from build123d import *

# Parameters (mm, degrees)
SKETCH8_W            = 23
SKETCH8_H            = 23
BOSS_EXTRUDE4_DEPTH  = 0.98
SKETCH16_W           = 9.9
SKETCH16_H           = 9.3
BOSS_EXTRUDE11_DEPTH = 0.84
BOSS_EXTRUDE11_TAPER = 20
SKETCH17_R           = 0.522081484
BOSS_EXTRUDE12_DEPTH = 0.1


with BuildPart() as part:
    # Sketch8 → Boss-Extrude4 (new body)
    with BuildSketch(Plane(origin=(0, 0, 0), x_dir=(1, 0, 0), z_dir=(0, 1, 0))):
        Rectangle(SKETCH8_W, SKETCH8_H)
    extrude(amount=BOSS_EXTRUDE4_DEPTH)

    # Sketch16 → Boss-Extrude11 (add)
    with BuildSketch(Plane(origin=(0, 0.98, 0), x_dir=(1, 0, 0), z_dir=(0, 1, 0))):
        Rectangle(SKETCH16_W, SKETCH16_H)
    extrude(amount=BOSS_EXTRUDE11_DEPTH, taper=BOSS_EXTRUDE11_TAPER)

    # Sketch17 → Boss-Extrude12 (add)
    with BuildSketch(Plane(origin=(0, 0.98, 0), x_dir=(1, 0, 0), z_dir=(0, 1, 0))):
        with Locations((-10.659163623, -10.593903438)):
            Circle(SKETCH17_R)
    extrude(amount=BOSS_EXTRUDE12_DEPTH)


solid = part.part
Can you work these out from the model? Positions are in its coordinate system, mm. A direction names the side the tool comes from. Coordinates: 2 decimals unless noted, no trailing zeros. Order: outer loops, then holes, each group sorted by start corner. A loop starts at its lowest first (then second) coordinate and runs counter-clockwise, first axis right, second up. Notation, with made-up numbers: (-19, 86) - (22, 86) arc R16 ccw to (22, 107) - close; hole circle Ø2 at (76.25, 50). An arc over 180 degrees is marked (long way). Answer as a JSON object with one key per item and string values. Group by question number.
Q1. Imagine slicing it at A-A (z = -5). Please give me the cut outline in (x, y).
Q2. Will these pins go through, and if not, where does the flat tip stop? P1, Ø8, axis at x = -9, z = -8, coming from the +Y side; P2, Ø0.8, axis at x = -10.5, z = 10.5, coming from the +Y side.
Q3. I need wall thicknesses on line 1 (Y direction, x = 10, z = -6); line 2 (X direction, y = 1.3, z = -4.5); line 3 (Z direction, x = 4, y = 1.3). Which ranges of each line are inside material? Lowest first, please. Write a range as from..to.
Q4. On a 3-axis mill with a long thin cutter (end or side, diameter ignored), from which of +Z, -Z, +X, -X, +Y, -Y can I reach the whole of each face in a straight line? I mean faces 1 (the face through (-10.7, 1.08, 10.6)), 2 (the face through (-5.3, 0.98, -0.2)). Say none if no direction works.
Q5. Imagine slicing it at B-B (x = 8.5). Please give me the cut outline in (y, z), and give its area (3 significant figures).
Determined:
{
 "1": {"outline": "(-11.5, 0) - (11.5, 0) - (11.5, 0.98) - (-11.5, 0.98) - close"},
 "2": {"P1": "stops at y = 0.98", "P2": "stops at y = 1.08"},
 "3": {"line 1": "y = 0..0.98", "line 2": "x = -4.83..4.83", "line 3": "z = -4.53..4.53"},
 "4": {"face 1": "+Z, -Z, +X, -X, +Y", "face 2": "+Y"},
 "5": {"outline": "(0, -11.5) - (0.98, -11.5) - (0.98, 11.5) - (0, 11.5) - close", "area": "22.5 mm2"}
}
